Model file for the job. Use its own axes, mm. Face numbers are marked on the shaded views. Give positions to 0.01 mm unless a question says otherwise; leave off trailing zeros. Order: outer loops, then holes, each group sorted by start corner. A loop starts at its lowest first (then second) coordinate and runs counter-clockwise, first axis right, second up. Notation, with made-up numbers: M -16.75,34.5 L 1.25,34.5 A20 ccw 1.25,63.5 Z; hole C -15,-22.75 d5. An arc over 180 degrees is marked long. Return JSON: item names as keys, results as strings. Group by question number.
1. Wall check: probe 1 along X at (y, z) = (1, 13.75); probe 2 along X at (y, z) = (1, 9). Give the ranges that are in metal, low to high. Write a range as [from, to].
2. Slice it at D-D on y = -16. List the corners of the cut face in (x, z).
3. Two-plate mould, pull along Y, no slides. Class the marked faces 1 and 2: released by +Y, released by -Y, zero draft, split by the parting line, or undercut.
4. Slice it at C-C on z = 12.5. List the corners of the cut face in (x, y).
5. Slice it at A-A on x = 0. List the corners of the cut face in (y, z), then the cut area to 3 significant figures.
6. Pin check, flat tips, straight feed: pin 1 (4 mm diameter, centred on x = -25, z = 12.5, fed in from -Y); pin 2 (4 mm diameter, centred on y = -7, z = 5.5, fed in from +X); pin 3 (6 mm diameter, centred on x = -18, z = 13, fed in from -Y). Stop position of each tip, or through.
7. Slice it at B-B on y = 0. List the corners of the cut face in (x, z), then the cut area to 3 significant figures.
from build123d import *

# Parameters (mm, degrees)
F0_R     = 42
F0_R_2   = 40.5
F1_DEPTH = 15
F3_R     = 3.5
F4_DEPTH = 7
F5_R     = 1


with BuildPart() as f1:
    # F0 (on Top) → F1 (new body)
    with BuildSketch(Plane.XY):
        Circle(F0_R)
        Circle(F0_R_2, mode=Mode.SUBTRACT)
    extrude(amount=F1_DEPTH)

    # F3 (on offset) → F4 (join)
    with BuildSketch(Plane.YZ.offset(41)):
        with Locations((0, 7.840633)):
            Circle(F3_R)
    extrude(amount=F4_DEPTH)

    # F5
    f5_edges = [f1.edges().sort_by_distance(p)[0] for p in [
        (48, -3.5, 7.840633),
    ]]
    fillet(f5_edges, radius=F5_R)


solid = f1.part
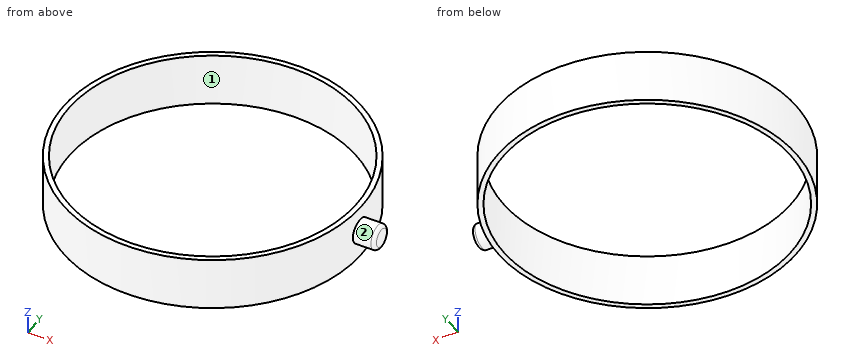
Result:
{
 "1": {"probe 1": "x = [-41.99, -40.49], [40.49, 41.99]", "probe 2": "x = [-41.99, -40.49], [40.49, 48]"},
 "2": {"outline": "M -38.83,0 L -37.21,0 L -37.21,15 L -38.83,15 Z; M 37.21,0 L 38.83,0 L 38.83,15 L 37.21,15 Z"},
 "3": {"face 1": "undercut", "face 2": "split by the parting line"},
 "4": {"outline": "C 0,0 d84; hole C 0,0 d81"},
 "5": {"outline": "M -42,0 L -40.5,0 L -40.5,15 L -42,15 Z; M 40.5,0 L 42,0 L 42,15 L 40.5,15 Z", "area": "45.0 mm2"},
 "6": {"pin 1": "stops at y = -35.14", "pin 2": "stops at x = 41.7", "pin 3": "stops at y = -39.23"},
 "7": {"outline": "M -42,0 L -40.5,0 L -40.5,15 L -42,15 Z; M 40.5,0 L 42,0 L 42,4.34 L 47,4.34 A1 ccw 48,5.34 L 48,10.34 A1 ccw 47,11.34 L 42,11.34 L 42,15 L 40.5,15 Z", "area": "86.6 mm2"}
}
